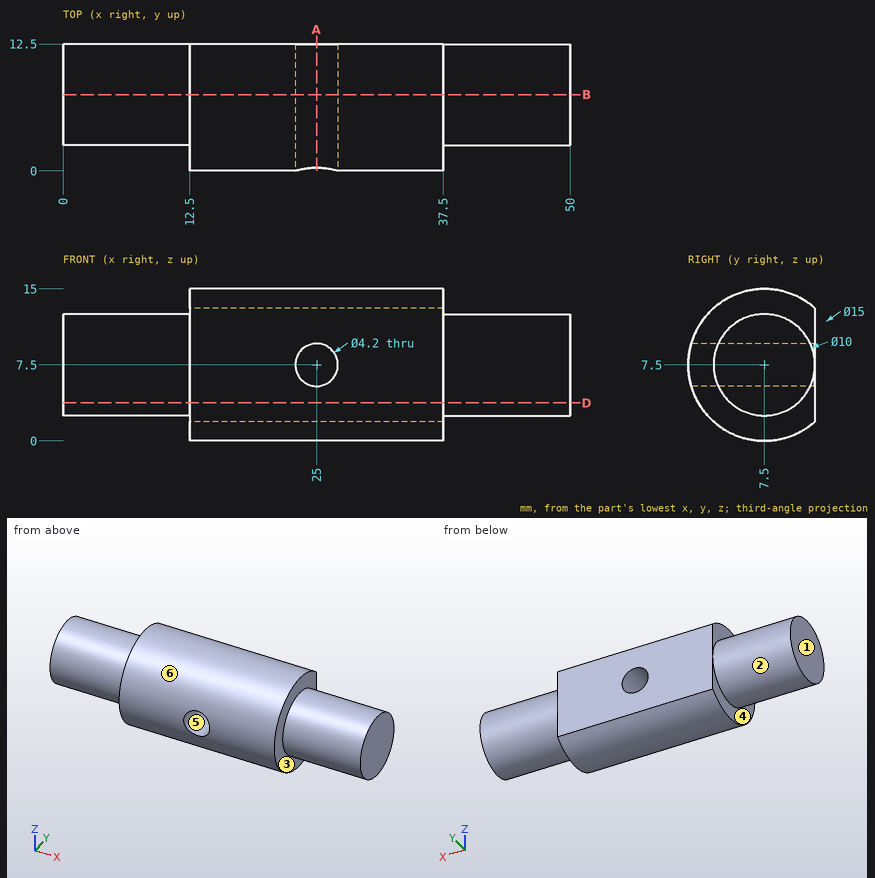
Print and shaded views of the part. All mm, measured from the part's lowest x, y and z. A direction names the side the tool comes from. Coordinates: 2 decimals unless noted, no trailing zeros. Order: outer loops, then holes, each group sorted by start corner. A loop starts at its lowest first (then second) coordinate and runs counter-clockwise, first axis right, second up.
(1) Slice it at A-A, the plane x = 25. Write the cut outline in (y, z), and give its area (3 significant figures).
Check sheet entries:
outline: (0.3, 5.4) arc R7.5 ccw to (12.5, 1.91) - (12.5, 5.4) - close; (0.3, 9.6) - (12.5, 9.6) - (12.5, 13.09) arc R7.5 ccw to start
area: 105 mm2
(2) Tool access for the marked faces 1, 2 and 3: list every direction of +Z, -Z, +X, -X, +Y, -Y with a clear straight run to the whole face (end or side of a thin tool).
Check sheet entries:
face 1: +Z, -Z, -X, +Y, -Y
face 2: -X
face 3: +X
(3) Slice it at B-B, the plane y = 7.5. Write the cut outline in (x, z).
Check sheet entries:
outline: (0, 2.5) - (12.5, 2.5) - (12.5, 0) - (37.5, 0) - (37.5, 2.5) - (50, 2.5) - (50, 12.5) - (37.5, 12.5) - (37.5, 15) - (12.5, 15) - (12.5, 12.5) - (0, 12.5) - close; hole circle Ø4.2 at (25, 7.5)
(4) Pull direction Z, two halves, no side cores. Call the marked faces 4, 5 and 6: pulls with the +Z half, pulls with the -Z half, needs draft (parallel to the pull), parting line crosses it, or undercut.
Check sheet entries:
face 4: needs draft
face 5: undercut
face 6: parting line crosses it
(5) Probe L1, parallel to Z at x = 25, y = 2.5; L2, parallel to X at y = 5.5, z = 1.25; L3, parallel to Z at x = 25, y = 5.5. List the from-to ranges inside material, lowest first.
Check sheet entries:
L1: z = 1.91 to 5.4, 9.6 to 13.09
L2: x = 12.5 to 37.5
L3: z = 0.27 to 5.4, 9.6 to 14.73
(6) Pin check, flat tips, straight feed: pin 1 Ø5 at (x, y) = (35, 10.5) entering from -Z; pin 2 Ø1 at (x, z) = (38.5, 5.5) entering from -Y; pin 3 Ø1.5 at (x, y) = (14, 1.5) entering from +Z; pin 4 Ø3 at (y, z) = (6, 4.5) entering from -X. Stop position of each tip, or through.
Check sheet entries:
pin 1: stops at z = 0.02
pin 2: stops at y = 2.73
pin 3: stops at z = 12.86
pin 4: stops at x = 0
(7) Slice it at D-D, the plane z = 3.75. Write the cut outline in (x, y), and give its area (3 significant figures).
Check sheet entries:
outline: (0, 4.19) - (12.5, 4.19) - (12.5, 1) - (37.5, 1) - (37.5, 4.19) - (50, 4.19) - (50, 10.81) - (37.5, 10.81) - (37.5, 12.5) - (12.5, 12.5) - (12.5, 10.81) - (0, 10.81) - close
area: 453 mm2
